For this review, take the finished solid that the model builds, in its own axes (mm). A direction names the side the tool comes from. Coordinates: 2 decimals unless noted, no trailing zeros. Write each loop counter-clockwise with the first axis right and the second up, starting at its lowest first coordinate (ties: lowest second). Pieces come first, ordered by that corner, then holes.
1) We need section A-A on x = 598.5. Write out the cut boundary in (y, z).
2) We need section B-B on y = 43. Write out the cut boundary in (x, z), then the cut area to 3 significant figures.
3) To check wall thickness, follow line 1 along Y through (x, z) = (69.85, -1); line 2 along Y through (x, z) = (277.5, 25); line 3 along Z through (x, y) = (475, 102). State the ranges of each line that lie inside material, in increasing order.
4) For faces 1 (the face through (370, 20.947, 19)), 2 (the face through (44.45, 35, -1)), 3 (the face through (704.85, 35, -1)), list the 3-axis set-ups (+Z, -Z, +X, -X, +Y, -Y) from which the entire face can be reached by the end or side of a thin tool; tool diameter is ignored.
5) Mouldability with a two-part tool opening along Y and no side actions: class faces 4 (the face through (0, 77.9, 13.1)), 5 (the face through (369, 64, 0)), 6 (the face through (21, 78.097, 19)), 7 (the face through (369, 107.95, 19)) as pulls with the +Y half, pulls with the -Y half, needs draft (parallel to the pull), parting line crosses it, or undercut.
6) Insertion check: P1, Ø1.5, axis at x = 374, z = 14, coming from the +Y side; P2, Ø12, axis at x = 214.5, y = 76, coming from the +Z side; P3, Ø9, axis at x = 374.65, z = 13.98, coming from the +Y side; P4, Ø11, axis at x = 733.42, z = 13.98, coming from the -Y side. Each pin has a flat end and moves straight along its axis. Give the tip position at first contact, or say it passes through.
from build123d import *

# Parameters (mm, degrees)
BASE_FLANGE1_DEPTH               = 1.89738
EDGE_FLANGE1_DEPTH               = 749.3
EDGE_FLANGE1_2_DEPTH             = 44.47667
EDGE_FLANGE1_START               = 704.82333
EDGE_FLANGE1_3_DEPTH             = 44.47667
EDGE_FLANGE1_START_2             = 43.52798
EDGE_FLANGE1_4_DEPTH             = 0.94869
EDGE_FLANGE1_5_DEPTH             = 0.94869
EDGE_FLANGE1_START_3             = 44.45
EDGE_FLANGE1_6_DEPTH             = 660.4
EDGE_FLANGE1_7_DEPTH             = 749.3
EDGE_FLANGE1_8_DEPTH             = 43.52798
EDGE_FLANGE1_START_4             = 705.77202
EDGE_FLANGE1_9_DEPTH             = 43.52798
FILLET1_R                        = 3.175
F_10_0_1935_DIAMETER_HOLE1_D     = 4.9149
F_17_64_0_26563_DIAMETER_HOLE2_D = 6.747002


# Read off the part's stored shape, not the designer's step: Edge-Flange1
# Sheet-metal steps are written as plain solids
with BuildPart() as part:
    # Sketch1 → Base-Flange1 (new body)
    with BuildSketch(Plane.XY):
        Polygon((44.45, 19.05), (704.85, 19.05), (704.85, 76.2), (749.3, 76.2), (749.3, 107.95), (0, 107.95), (0, 76.2), (44.45, 76.2), align=None)
    extrude(amount=-BASE_FLANGE1_DEPTH)

    # Edge-Flange1 outline → Edge-Flange1 (cut)
    with BuildSketch(Plane.YZ):
        with BuildLine():
            Line((19.05, -1.89738), (23.48738, -1.89738))
            ThreePointArc((23.48738, -1.89738), (21.435625133, -1.394544857), (19.84887189, 0))
            Line((19.84887189, 0), (19.05, 0))
            Line((19.05, 0), (19.05, -1.89738))
        make_face()
        with BuildLine():
            ThreePointArc((107.15112811, 0), (105.564374867, -1.394544857), (103.51262, -1.89738))
            Line((103.51262, -1.89738), (107.95, -1.89738))
            Line((107.95, -1.89738), (107.95, 0))
            Line((107.95, 0), (107.15112811, 0))
        make_face()
    extrude(amount=EDGE_FLANGE1_DEPTH, mode=Mode.SUBTRACT)

    # Edge-Flange1 2 outline → Edge-Flange1 2 (cut)
    with BuildSketch(Plane.YZ):
        with BuildLine():
            Line((76.2, 0), (76.2, -1.89738))
            Line((76.2, -1.89738), (80.63738, -1.89738))
            ThreePointArc((80.63738, -1.89738), (78.585625133, -1.394544857), (76.99887189, 0))
            Line((76.99887189, 0), (76.2, 0))
        make_face()
    extrude(amount=EDGE_FLANGE1_2_DEPTH, mode=Mode.SUBTRACT)

    # Edge-Flange1 3 outline → Edge-Flange1 3 (cut)
    with BuildSketch(Plane.YZ.offset(EDGE_FLANGE1_START)):
        with BuildLine():
            Line((76.2, 0), (76.2, -1.89738))
            Line((76.2, -1.89738), (80.63738, -1.89738))
            ThreePointArc((80.63738, -1.89738), (78.585625133, -1.394544857), (76.99887189, 0))
            Line((76.99887189, 0), (76.2, 0))
        make_face()
    extrude(amount=EDGE_FLANGE1_3_DEPTH, mode=Mode.SUBTRACT)

    # Edge-Flange1 4 outline → Edge-Flange1 4 (cut)
    with BuildSketch(Plane.YZ.offset(EDGE_FLANGE1_START_2)):
        with BuildLine():
            ThreePointArc((76.99887189, 0), (78.585625133, -1.394544857), (80.63738, -1.89738))
            Line((80.63738, -1.89738), (81.58607, -1.89738))
            Line((81.58607, -1.89738), (81.58607, 0))
            Line((81.58607, 0), (76.99887189, 0))
        make_face()
    extrude(amount=EDGE_FLANGE1_4_DEPTH, mode=Mode.SUBTRACT)

    # Edge-Flange1 5 outline → Edge-Flange1 5 (cut)
    with BuildSketch(Plane.YZ.offset(EDGE_FLANGE1_START)):
        with BuildLine():
            ThreePointArc((76.99887189, 0), (78.585625133, -1.394544857), (80.63738, -1.89738))
            Line((80.63738, -1.89738), (81.58607, -1.89738))
            Line((81.58607, -1.89738), (81.58607, 0))
            Line((81.58607, 0), (76.99887189, 0))
        make_face()
    extrude(amount=EDGE_FLANGE1_5_DEPTH, mode=Mode.SUBTRACT)

    # Edge-Flange1 6 outline → Edge-Flange1 6 (add)
    with BuildSketch(Plane.YZ.offset(EDGE_FLANGE1_START_3)):
        with BuildLine():
            Line((19.84887189, 0), (23.48738, 0))
            ThreePointArc((23.48738, 0), (21.691328776, 0.743948776), (20.94738, 2.54))
            Line((20.94738, 2.54), (20.94738, 36.20262))
            Line((20.94738, 36.20262), (19.05, 36.20262))
            Line((19.05, 36.20262), (19.05, 2.54))
            ThreePointArc((19.05, 2.54), (19.254426871, 1.20866643), (19.84887189, 0))
        make_face()
        with BuildLine():
            ThreePointArc((106.05262, 2.54), (105.308671224, 0.743948776), (103.51262, 0))
            Line((103.51262, 0), (107.15112811, 0))
            ThreePointArc((107.15112811, 0), (107.745573129, 1.20866643), (107.95, 2.54))
            Line((107.95, 2.54), (107.95, 36.20262))
            Line((107.95, 36.20262), (106.05262, 36.20262))
            Line((106.05262, 36.20262), (106.05262, 2.54))
        make_face()
    extrude(amount=EDGE_FLANGE1_6_DEPTH)

    # Edge-Flange1 7 outline → Edge-Flange1 7 (add)
    with BuildSketch(Plane.YZ):
        with BuildLine():
            ThreePointArc((106.05262, 2.54), (105.308671224, 0.743948776), (103.51262, 0))
            Line((103.51262, 0), (107.15112811, 0))
            ThreePointArc((107.15112811, 0), (107.745573129, 1.20866643), (107.95, 2.54))
            Line((107.95, 2.54), (107.95, 36.20262))
            Line((107.95, 36.20262), (106.05262, 36.20262))
            Line((106.05262, 36.20262), (106.05262, 2.54))
        make_face()
    extrude(amount=EDGE_FLANGE1_7_DEPTH)

    # Edge-Flange1 8 outline → Edge-Flange1 8 (add)
    with BuildSketch(Plane.YZ):
        with BuildLine():
            ThreePointArc((76.2, 2.54), (76.404426871, 1.20866643), (76.99887189, 0))
            Line((76.99887189, 0), (80.63738, 0))
            ThreePointArc((80.63738, 0), (78.841328776, 0.743948776), (78.09738, 2.54))
            Line((78.09738, 2.54), (78.09738, 36.20262))
            Line((78.09738, 36.20262), (76.2, 36.20262))
            Line((76.2, 36.20262), (76.2, 2.54))
        make_face()
    extrude(amount=EDGE_FLANGE1_8_DEPTH)

    # Edge-Flange1 9 outline → Edge-Flange1 9 (add)
    with BuildSketch(Plane.YZ.offset(EDGE_FLANGE1_START_4)):
        with BuildLine():
            ThreePointArc((76.2, 2.54), (76.404426871, 1.20866643), (76.99887189, 0))
            Line((76.99887189, 0), (80.63738, 0))
            ThreePointArc((80.63738, 0), (78.841328776, 0.743948776), (78.09738, 2.54))
            Line((78.09738, 2.54), (78.09738, 36.20262))
            Line((78.09738, 36.20262), (76.2, 36.20262))
            Line((76.2, 36.20262), (76.2, 2.54))
        make_face()
    extrude(amount=EDGE_FLANGE1_9_DEPTH)

    # Fillet1
    fillet1_edges = [part.edges().sort_by_distance(p)[0] for p in [
        (749.3, 107.00131, 36.20262),
        (0, 107.00131, 36.20262),
        (0, 77.14869, 36.20262),
        (44.45, 19.99869, 36.20262),
        (704.85, 19.99869, 36.20262),
        (749.3, 77.14869, 36.20262),
    ]]
    fillet(fillet1_edges, radius=FILLET1_R)

    # #10 (0.1935) Diameter Hole1 (through all)
    with Locations(Plane(origin=(0, 0, -1.89738), x_dir=(-1, 0, 0), z_dir=(0, 0, -1))):
        with Locations((-679.45, 53.975), (-631.825, 53.975), (-117.475, 53.975), (-69.85, 53.975)):
            Hole(F_10_0_1935_DIAMETER_HOLE1_D / 2)

    # 17/64 (0.26563) Diameter Hole2 (through all)
    with Locations(Plane(origin=(0, 107.95, 0), x_dir=(1, 0, 0), z_dir=(0, 1, 0))):
        with Locations((733.425, -13.97762), (374.65, -13.97762), (15.875, -13.97762)):
            Hole(F_17_64_0_26563_DIAMETER_HOLE2_D / 2)


solid = part.part
Result:
1. outline: (19.05, 2.54) arc R4.44 ccw to (23.49, -1.9) - (103.51, -1.9) arc R4.44 ccw to (107.95, 2.54) - (107.95, 36.2) - (106.05, 36.2) - (106.05, 2.54) arc R2.54 cw to (103.51, 0) - (23.49, 0) arc R2.54 cw to (20.95, 2.54) - (20.95, 36.2) - (19.05, 36.2) - close
2. outline: (44.45, -1.9) - (704.85, -1.9) - (704.85, 0) - (44.45, 0) - close
2. area: 1,250 mm2
3. line 1: y = 20.81 to 51.52, 56.43 to 106.19
3. line 2: y = 19.05 to 20.95, 106.05 to 107.95
3. line 3: z = -1.9 to 0
4. face 1: +Z, +X, -X
4. face 2: +Z, -Z, -X, -Y
4. face 3: +Z, -Z, +X, -Y
5. face 4: needs draft
5. face 5: undercut
5. face 6: undercut
5. face 7: pulls with the +Y half
6. P1: passes through
6. P2: stops at z = 0
6. P3: stops at y = 107.95
6. P4: stops at y = 76.2
